```python
from build123d import *
from OCP.BRepFilletAPI import BRepFilletAPI_MakeFillet

# Parameters (mm, degrees)
BOSS_EXTRUDE1_DEPTH      = 6
BOSS_EXTRUDE2_DEPTH      = 2.15
BOSS_EXTRUDE2_DEPTH_BACK = 1.5
SKETCH3_W                = 18.5
SKETCH3_H                = 3.5
SKETCH4_W                = 15.5
SKETCH4_H                = 1.35
CUT_EXTRUDE1_DEPTH       = 2.5
CUT_EXTRUDE2_REACH       = 24.817
SKETCH5_W                = 9.5
SKETCH5_H                = 5
FILLET1_R                = 0.65
SKETCH6_R                = 1.9
BOSS_EXTRUDE3_DEPTH      = 2
BOSS_EXTRUDE4_DEPTH      = 1.17
BOSS_EXTRUDE4_DEPTH_BACK = 1
SKETCH7_R                = 1.9
FILLET2_R1               = 1
FILLET2_R2               = 2


with BuildPart() as part:
    # Sketch2 → Boss-Extrude1 (new body)
    with BuildSketch(Plane(origin=(0, 0, 0), x_dir=(0, 0, -1), z_dir=(1, 0, 0))):
        with BuildLine():
            Line((0, 0), (18.9, 0))
            Line((18.9, 0), (18.9, 3.5))
            Line((18.9, 3.5), (17.25, 3.5))
            ThreePointArc((17.25, 3.5), (17.002512627, 3.397487373), (16.9, 3.15))
            Line((16.9, 3.15), (16.9, 3))
            Line((16.9, 3), (17.5, 2.4))
            Line((17.5, 2.4), (17.5, 1.5))
            Line((17.5, 1.5), (0, 1.5))
            Line((0, 1.5), (0, 0))
        make_face()
    extrude(amount=BOSS_EXTRUDE1_DEPTH)

    # Sketch3 → Boss-Extrude2 (add, two sides: drawn at the far end of the back side and taken through both)
    with BuildSketch(Plane(origin=(0, 1.5, 0), x_dir=(1, 0, 0), z_dir=(0, 1, 0)).offset(-BOSS_EXTRUDE2_DEPTH_BACK)):
        with Locations((3, 0.25)):
            Rectangle(SKETCH3_W, SKETCH3_H)
    extrude(amount=BOSS_EXTRUDE2_DEPTH + BOSS_EXTRUDE2_DEPTH_BACK)

    # Sketch4 → Cut-Extrude1 (cut)
    with BuildSketch(Plane(origin=(0, 0, -2), x_dir=(-1, 0, 0), z_dir=(0, 0, -1))):
        with Locations((-3, 2.175)):
            Rectangle(SKETCH4_W, SKETCH4_H)
    extrude(amount=-CUT_EXTRUDE1_DEPTH, mode=Mode.SUBTRACT)

    # Cut-Extrude2: up to this face of the body (flat: up to its plane)
    cut_extrude2_end = Plane(part.part.faces().sort_by_distance((3, 1.5, -7.102941176))[0])
    # Sketch5 → Cut-Extrude2 (cut, up to the picked face)
    with BuildSketch(Plane(origin=(0, 3.65, 0), x_dir=(1, 0, 0), z_dir=(0, 1, 0)), mode=Mode.PRIVATE) as cut_extrude2_sk1:
        with Locations((3, 1)):
            Rectangle(SKETCH5_W, SKETCH5_H)
    cut_extrude2_tool1 = split(extrude(cut_extrude2_sk1.sketch, amount=-CUT_EXTRUDE2_REACH, mode=Mode.PRIVATE), bisect_by=cut_extrude2_end, keep=Keep.BOTH, mode=Mode.PRIVATE)
    add(cut_extrude2_tool1.solids().sort_by(Axis((3, 3.65, -1), (0, -1, 0)))[0], mode=Mode.SUBTRACT)

    # Fillet1
    fillet1_edges = [part.edges().sort_by_distance(p)[0] for p in [
        (-3.25, 2.85, -2),
        (9.25, 2.85, -2),
    ]]
    fillet(fillet1_edges, radius=FILLET1_R)

    # Sketch6 → Boss-Extrude3 (add)
    with BuildSketch(Plane.XY.offset(1.5)):
        with BuildLine():
            Line((-5.4, 0), (6.4, 0))
            Line((6.4, 0), (6.4, -11))
            ThreePointArc((6.4, -11), (3, -14.4), (-0.4, -11))
            Line((-0.4, -11), (-5.4, -11))
            Line((-5.4, -11), (-5.4, 0))
        make_face()
        with Locations((3, -11)):
            Circle(SKETCH6_R, mode=Mode.SUBTRACT)
    extrude(amount=-BOSS_EXTRUDE3_DEPTH)

    # Sketch7 → Boss-Extrude4 (add, two sides: drawn at the far end of the back side and taken through both)
    with BuildSketch(Plane.ZY.offset(6.25).offset(-BOSS_EXTRUDE4_DEPTH_BACK)):
        with BuildLine():
            Line((1.5, 3.65), (-12.3, 3.65))
            Line((-12.3, 3.65), (-12.3, -11))
            ThreePointArc((-12.3, -11), (-8.9, -14.4), (-5.5, -11))
            Line((-5.5, -11), (1.5, -11))
            Line((1.5, -11), (1.5, 3.65))
        make_face()
        with Locations(Location((-8.9, -11, 0), (0, 0, 180))):
            Circle(SKETCH7_R, mode=Mode.SUBTRACT)
    extrude(amount=BOSS_EXTRUDE4_DEPTH + BOSS_EXTRUDE4_DEPTH_BACK)

    # Fillet2: one fillet with a radius per group of edges: ONE call of the kernel's fillet builder (fillet() takes one radius for all edges)
    fillet2_edges_1 = [part.edges().sort_by_distance(p)[0] for p in [
        (-7.42, -3.675, 1.5),
    ]]
    fillet2_edges_2 = [part.edges().sort_by_distance(p)[0] for p in [
        (6.4, 0, 0.5),
    ]]
    fillet2 = BRepFilletAPI_MakeFillet(part.part.solid().wrapped)
    for e in fillet2_edges_1:
        fillet2.Add(FILLET2_R1, e.wrapped)
    for e in fillet2_edges_2:
        fillet2.Add(FILLET2_R2, e.wrapped)
    add(Compound.cast(fillet2.Shape()), mode=Mode.REPLACE)


solid = part.part
```
Geometry: final body of the model. Coordinates: model frame, mm. A direction names the side the tool comes from. Round coordinates to 2 decimals unless told otherwise and drop trailing zeros. Loops run counter-clockwise (first coordinate to the right, second up) from the corner with the lowest first, then second, coordinate; pieces in that order, holes last. Notation, with made-up numbers: (42.25, 14) -> (63.25, 14) arc R25 ccw to (63.25, 53) -> close; hole circle Ø7 at (-1, 58.5). An arc over 180 degrees is marked (long way). Write each question's results on one line, items separated by ' | '.
Item 1: Cut plane B-B on y = -7.25. Return the cut outline in (x, z), and give its area (3 significant figures).
Answers below:
outline: (-7.42, -12.3) -> (-5.25, -12.3) -> (-5.25, -0.5) -> (6.4, -0.5) -> (6.4, 1.5) -> (-6.42, 1.5) arc R1 ccw to (-7.42, 0.5) -> close | area: 53.0 mm²
Item 2: Pull-direction query (Y, two-part tool) for faces 1 (the face through (3.1, -14.4, 0.5)), 2 (the face through (-6, -4, -12.3)), 3 (the face through (10.75, 2, -1)); classes: pulls with the +Y half, pulls with the -Y half, needs draft (parallel to the pull), parting line crosses it, or undercut.
Answers below:
face 1: pulls with the -Y half | face 2: needs draft | face 3: undercut
Item 3: Cut plane C-C on x = 3. Return the cut outline in (y, z), and give its area (3 significant figures).
Answers below:
outline: (-14.4, -0.5) -> (-12.9, -0.5) -> (-12.9, 1.5) -> (-14.4, 1.5) -> close; (-9.1, -0.5) -> (0, -0.5) -> (0, -18.9) -> (3.5, -18.9) -> (3.5, -17.25) arc R0.35 ccw to (3.15, -16.9) -> (3, -16.9) -> (2.4, -17.5) -> (1.5, -17.5) -> (1.5, 1.5) -> (-9.1, 1.5) -> close | area: 55.1 mm²
Item 4: Pin query (flat end, axial travel): pin 1 Ø3 at (x, z) = (-3.5, -11.5) entering from +Y; pin 2 Ø5 at (y, z) = (-6, -11) entering from +X; pin 3 Ø3.5 at (x, z) = (-4.5, -3) entering from -Y; pin 4 Ø8 at (x, y) = (9.5, -11) entering from -Z. Return the tip coordinate at first contact, or that it passes through.
Answers below:
pin 1: passes through | pin 2: stops at x = -5.25 | pin 3: stops at y = -11 | pin 4: stops at z = -0.5
Item 5: Cut plane D-D on x = -3.5. Return the cut outline in (y, z).
Answers below:
outline: (-11, -0.5) -> (0, -0.5) -> (0, -2) -> (1.5, -2) -> (1.5, 0.5) -> (2.85, 0.5) -> (2.85, -1.35) arc R0.65 ccw to (3.5, -2) -> (3.65, -2) -> (3.65, 1.5) -> (-11, 1.5) -> close
Item 6: Cut plane A-A on z = -8.9. Return the cut outline in (x, y).
Answers below:
outline: (-7.42, -14.4) -> (-5.25, -14.4) -> (-5.25, -12.9) -> (-7.42, -12.9) -> close; (-7.42, -9.1) -> (-5.25, -9.1) -> (-5.25, 3.65) -> (-7.42, 3.65) -> close; (0, 0) -> (6, 0) -> (6, 1.5) -> (0, 1.5) -> close
Item 7: Line query: probe 1 along Y at (x, z) = (-5.5, -8.75); probe 2 along Y at (x, z) = (3, 0.75); probe 3 along Y at (x, z) = (-6.5, 0). Output: solid intervals per line, ascending. Write a range as [from, to].
Answers below:
probe 1: y = [-14.4, -12.89], [-9.11, 3.65] | probe 2: y = [-14.4, -12.9], [-9.1, 1.5] | probe 3: y = [-11, 3.65]
Item 8: Set-up query: faces 4 (the face through (2, -5, -0.5)), 5 (the face through (-3, 2.85, 0)), 6 (the face through (0, 1, -10)), 7 (the face through (10, 1, -2)). Return all of +Z, -Z, +X, -X, +Y, -Y with unobstructed straight access to the full face (end or side cutting, diameter ignored); none if empty.
Answers below:
face 4: -Z, +X, -Y | face 5: -Z | face 6: -Z, +Y, -Y | face 7: -Z, +X, +Y, -Y
